Autodesk Fusion 360 part; units mm, degrees
sketch "Sketch2" plane through (0, 0, 0) normal (0, 1, 0) x (1, 0, 0)
  line L0 (0, -50) -> (80, -50)
  line L1 (0, -50) -> (-80, -50)
  line L2 (-80, -52.8) -> (80, -52.8)
  circle A0 centre (70, -50) radius 3.3
  circle A1 centre (-70, -50) radius 3.25
  line L3 (-70, -65) -> (70, -65)
  arc A2 (70, -65) -> (70, -35) centre (70, -50) ccw
  line L4 (70, -35) -> (-70, -35)
  arc A3 (-70, -35) -> (-70, -65) centre (-70, -50) ccw
  line L5 (-70, -50) -> (70, -50) construction
  ellipse E0 centre (0, -50) end of major axis (52.5047, -50) minor radius 10
  line L6 (-52.5047, -50) -> (52.5047, -50)
  line L7 (0, -60) -> (0, -40)
  circle A4 centre (-70, -50) radius 0.75
  circle A5 centre (70, -50) radius 0.75
  dimension "d7" = 80
  dimension "d8" = 80
  dimension "d9" = 2.8
  dimension "d10" = 6.6
  dimension "d11" = 6.5
  dimension "d12" = 30
  dimension "d13" = 20
  dimension "d14" = 1.5
  dimension "d15" = 1.5
extrude "Extrude1" add sketch "Sketch2" along normal blind 10 contours L0 L2 A0 E0 | L1 L2 A1 E0 | L0 A0 A5 | L0 L2 A0 A5 | L1 L2 A1 A4 | L1 A1 A4 | L0 A5 | L0 A5 | L2 A0 | L1 A4 | L1 A4 | L2 A1 | L3 A2 L4 A3
extrude "Extrude2" cut sketch "Sketch2" along normal blind 7 contours L0 A0 A5 | L0 L2 A0 A5 | L1 L2 A1 A4 | L1 A1 A4
extrude "Extrude3" cut sketch "Sketch2" along normal blind 3 contours L0 A5 | L0 A5 | L1 A4 | L1 A4
The listing builds one solid part. Answer for the finished solid, in the listing's coordinates (mm). A direction names the side the tool comes from. Round coordinates to 2 decimals unless told otherwise and drop trailing zeros. Put each result on its own line as item: value. Start each with the question number.
(1) For faces 1 (the flat face through (-70, 3, 52.8)), 2 (the flat face through (1, 5, 35)), determine the directions among +Z, -Z, +X, -X, +Y, -Y from which every point of the face is accessible in a straight line to the end or side of a thin tool.
(2) Find section A-A (y = 4.75). State how many separate pieces and enclosed holes the cut face has, plus the area to 3 significant figures.
(3) Straight lines are drawn through the part: probe 1 along Z at (x, y) = (-70, 3.75); probe 2 along X at (y, z) = (4.25, 50); probe 3 along Z at (x, y) = (70, 4.5). For each, find the intervals that lie inside material, in ascending order. Write a range as from..to.
(4) Given P1, Ø6, axis at y = 7, z = 60.5, coming from the -X side; P2, Ø3, axis at x = -69, z = 49.5, coming from the -Y side, each flat-ended and moving along its own axis, determine where each tip first touches the part or whether it passes through.
(5) Determine the mould class of faces 3 (the flat face through (70, 3, 52.8)), 4 (the flat face through (-1, 5, 65)), 5 (the cylindrical face through (-85, 5, 50)), 6 (the cylindrical face through (-70.119, 3.451, 46.752)) for opening direction X: released by +X, released by -X, zero draft, split by the parting line, or undercut.
Reply:
1. face 1: -Y
1. face 2: -Z, +X, -X, +Y, -Y
2. separate pieces: 3
2. enclosed holes: 3
2. area: 3,200 mm^2
3. probe 1: 35..46.75, 49.25..50.75, 52.8..65
3. probe 2: -85..-73.25, -70.75..-69.25, -66.75..-52.5, 52.5..66.7, 69.25..70.75, 73.3..85
3. probe 3: 35..46.7, 49.25..50.75, 52.8..65
4. P1: x = -82.99
4. P2: y = 3
5. face 3: undercut
5. face 4: zero draft
5. face 5: released by -X
5. face 6: undercut
